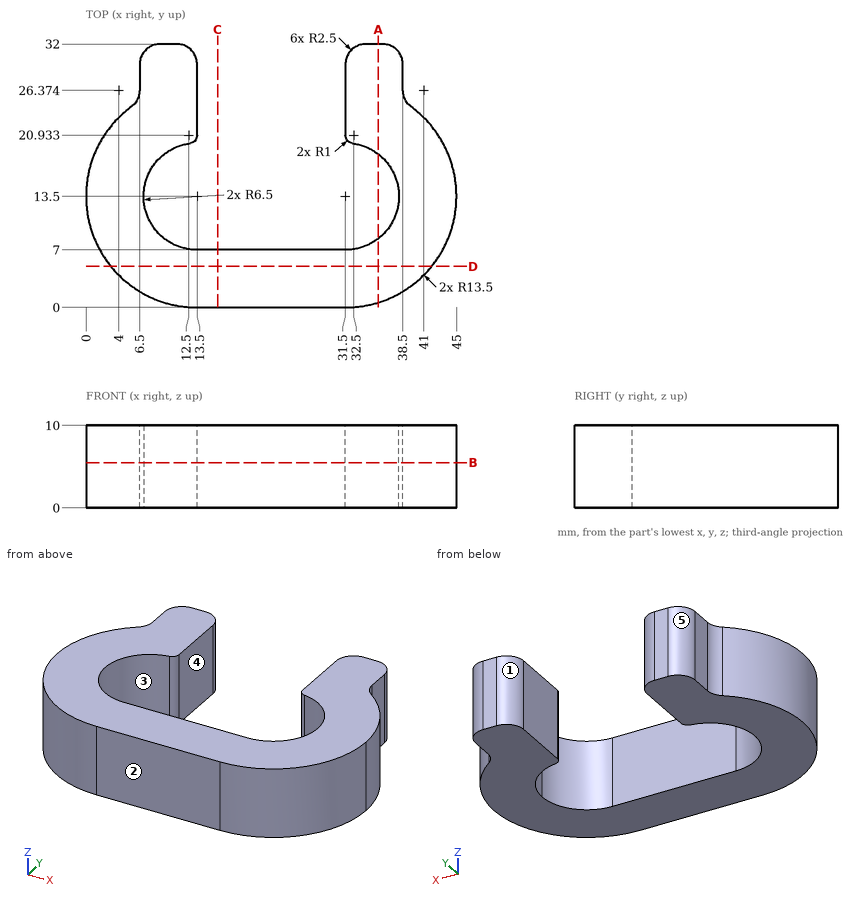
Geometry: see drawing. Coordinates: mm, zero at the bounding-box minimum. A direction names the side the tool comes from. Coordinates: 2 decimals unless noted, no trailing zeros. Order: outer loops, then holes, each group sorted by start corner. A loop starts at its lowest first (then second) coordinate and runs counter-clockwise, first axis right, second up. Notation, with made-up numbers: M 53.5,1 L 97.5,1 A5 cw 97.5,6 Z; hole C -8,-36.5 d11. An arc over 180 degrees is marked long. Answer in a Markdown table with one row per item. Add a question column.
Q1. Section query C-C on x = 16. Return the cut outline in (y, z), and give its area (3 significant figures).
Q2. Reachability of the marked faces 4 and 5 from +Z, -Z, +X, -X, +Y, -Y: full face, straight path, thin tool, end or side. Return the list, or none.
Q3. Section query B-B on z = 5.5. Return the cut outline in (x, y) (1 decimal).
Q4. Section query A-A on x = 35.5. Return the cut outline in (y, z).
Q5. Mould query, pull axis Y, two halves, no side actions, for the marked faces 1, 2 and 3. Classes: released by +Y, released by -Y, zero draft, split by the parting line, or undercut.
Q6. Line query: L1, parallel to X at y = 27.5, z = 3.25; L2, parallel to X at y = 17, z = 6.25; L3, parallel to Y at x = 18.5, z = 9.5. Output: solid intervals per line, ascending.
Q7. Contact query for flat-ended pins moving along their axis: P1, Ø5, axis at x = 26.5, z = 7.5, coming from the +Y side; P2, Ø4, axis at y = 10.5, z = 7, coming from the +X side; P3, Ø1, axis at x = 13.5, z = 4.5, coming from the +Y side. Output: stop coordinate, or through.
Q8. Section query D-D on y = 5. Return the cut outline in (x, z).
Completed:
| question | item | result |
|---|---|---|
| 1 | outline | M 0,0 L 7,0 L 7,10 L 0,10 Z |
| 1 | area | 70.0 mm2 |
| 2 | face 4 | +Z, -Z, +Y |
| 2 | face 5 | +Z, -Z, -X, +Y |
| 3 | outline | M 5.5,24.4 A13.5 ccw 13.5,0 L 31.5,0 A13.5 ccw 39.5,24.4 A2.5 cw 38.5,26.4 L 38.5,29.5 A2.5 ccw 36,32 L 34,32 A2.5 ccw 31.5,29.5 L 31.5,20.9 A1 ccw 32.4,19.9 A6.5 cw 31.5,7 L 13.5,7 A6.5 cw 12.6,19.9 A1 ccw 13.5,20.9 L 13.5,29.5 A2.5 ccw 11,32 L 9,32 A2.5 ccw 6.5,29.5 L 6.5,26.4 A2.5 cw Z |
| 4 | outline | M 0.61,0 L 8.38,0 L 8.38,10 L 0.61,10 Z; M 18.62,0 L 32,0 L 32,10 L 18.62,10 Z |
| 5 | face 1 | released by +Y |
| 5 | face 2 | released by -Y |
| 5 | face 3 | undercut |
| 6 | L1 | x = 6.5 to 13.5, 31.5 to 38.5 |
| 6 | L2 | x = 0.46 to 8.02, 36.98 to 44.54 |
| 6 | L3 | y = 0 to 7 |
| 7 | P1 | stops at y = 7 |
| 7 | P2 | stops at x = 44.96 |
| 7 | P3 | stops at y = 31 |
| 8 | outline | M 3.01,0 L 41.99,0 L 41.99,10 L 3.01,10 Z |
